Build history of the part. All positions in model axes, mm. Face numbers are marked on the shaded views. A direction names the side the tool comes from. Round coordinates to 2 decimals unless told otherwise and drop trailing zeros. Order: outer loops, then holes, each group sorted by start corner. A loop starts at its lowest first (then second) coordinate and runs counter-clockwise, first axis right, second up. Notation, with made-up numbers: (-32, -16) -> (-25, -16) arc R19 ccw to (-25, 4) -> close; hole circle Ø6 at (-13, 34). An arc over 180 degrees is marked (long way). Write item = value, one per line.
from build123d import *

# Parameters (mm, degrees)
SKETCH1_R           = 0.8
SKETCH1_W           = 15.5
SKETCH1_H           = 10.5
BOSS_EXTRUDE1_DEPTH = 3.8
SKETCH2_R           = 0.8
SKETCH2_W           = 4
SKETCH2_H           = 10.5
BOSS_EXTRUDE2_DEPTH = 1


with BuildPart() as part:
    # Sketch1 → Boss-Extrude1 (new body)
    with BuildSketch(Plane(origin=(0, 0, 0), x_dir=(1, 0, 0), z_dir=(0, 1, 0))):
        with BuildLine():
            Line((-7.75, 6), (7.75, 6))
            ThreePointArc((7.75, 6), (8.62532777, 5.798277313), (9.324082071, 5.233801294))
            Line((9.324082071, 5.233801294), (12.217602589, 1.542251618))
            ThreePointArc((12.217602589, 1.542251618), (12.75, 0), (12.217602589, -1.542251618))
            Line((12.217602589, -1.542251618), (9.324082071, -5.233801294))
            ThreePointArc((9.324082071, -5.233801294), (8.62532777, -5.798277313), (7.75, -6))
            Line((7.75, -6), (-7.75, -6))
            ThreePointArc((-7.75, -6), (-8.62532777, -5.798277313), (-9.324082071, -5.233801294))
            Line((-9.324082071, -5.233801294), (-12.217602589, -1.542251618))
            ThreePointArc((-12.217602589, -1.542251618), (-12.75, 0), (-12.217602589, 1.542251618))
            Line((-12.217602589, 1.542251618), (-9.324082071, 5.233801294))
            ThreePointArc((-9.324082071, 5.233801294), (-8.62532777, 5.798277313), (-7.75, 6))
        make_face()
        with Locations((10.25, 0)):
            Circle(SKETCH1_R, mode=Mode.SUBTRACT)
        with Locations((-10.25, 0)):
            Circle(SKETCH1_R, mode=Mode.SUBTRACT)
        Rectangle(SKETCH1_W, SKETCH1_H, mode=Mode.SUBTRACT)
    extrude(amount=BOSS_EXTRUDE1_DEPTH)

    # Sketch2 → Boss-Extrude2 (add)
    with BuildSketch(Plane(origin=(0, 3.8, 0), x_dir=(1, 0, 0), z_dir=(0, 1, 0))):
        with BuildLine():
            Line((-9.324082071, 5.233801294), (-12.217602589, 1.542251618))
            ThreePointArc((-12.217602589, 1.542251618), (-12.75, 0), (-12.217602589, -1.542251618))
            Line((-12.217602589, -1.542251618), (-9.324082071, -5.233801294))
            ThreePointArc((-9.324082071, -5.233801294), (-8.62532777, -5.798277313), (-7.75, -6))
            Line((-7.75, -6), (7.75, -6))
            ThreePointArc((7.75, -6), (8.62532777, -5.798277313), (9.324082071, -5.233801294))
            Line((9.324082071, -5.233801294), (12.217602589, -1.542251618))
            ThreePointArc((12.217602589, -1.542251618), (12.75, 0), (12.217602589, 1.542251618))
            Line((12.217602589, 1.542251618), (9.324082071, 5.233801294))
            ThreePointArc((9.324082071, 5.233801294), (8.62532777, 5.798277313), (7.75, 6))
            Line((7.75, 6), (-7.75, 6))
            ThreePointArc((-7.75, 6), (-8.62532777, 5.798277313), (-9.324082071, 5.233801294))
        make_face()
        with Locations((10.25, 0)):
            Circle(SKETCH2_R, mode=Mode.SUBTRACT)
        with Locations((-10.25, 0)):
            Circle(SKETCH2_R, mode=Mode.SUBTRACT)
        with Locations((5.75, 0)):
            Rectangle(SKETCH2_W, SKETCH2_H, mode=Mode.SUBTRACT)
    extrude(amount=BOSS_EXTRUDE2_DEPTH)


solid = part.part
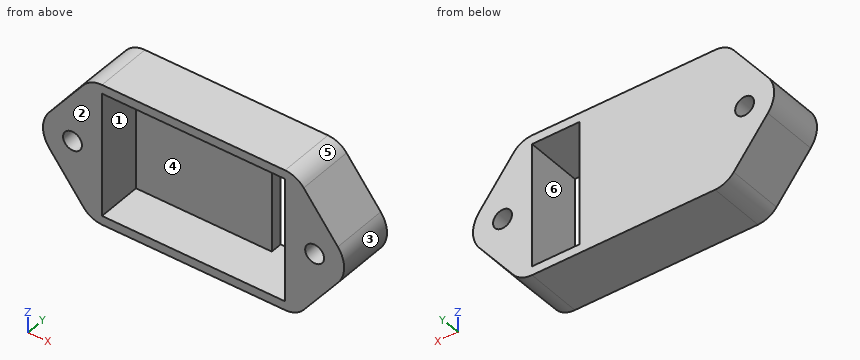
Q1. Cut at D-D, the plane z = 2.25. List the corners of the cut face in (x, y).
Check values:
outline = (-11.66, 0) -> (-7.75, 0) -> (-7.75, 3.8) -> (3.75, 3.8) -> (3.75, 4.8) -> (-11.66, 4.8) -> close; (7.75, 0) -> (11.66, 0) -> (11.66, 4.8) -> (7.75, 4.8) -> close
Q2. Cut at B-B, the plane y = 2.4. List the corners of the cut face in (x, z).
Check values:
outline = (-12.22, -1.54) -> (-9.32, -5.23) arc R2 ccw to (-7.75, -6) -> (7.75, -6) arc R2 ccw to (9.32, -5.23) -> (12.22, -1.54) arc R2.5 ccw to (12.22, 1.54) -> (9.32, 5.23) arc R2 ccw to (7.75, 6) -> (-7.75, 6) arc R2 ccw to (-9.32, 5.23) -> (-12.22, 1.54) arc R2.5 ccw to start; hole circle Ø1.6 at (-10.25, 0); hole (-7.75, -5.25) -> (7.75, -5.25) -> (7.75, 5.25) -> (-7.75, 5.25) -> close; hole circle Ø1.6 at (10.25, 0)
Q3. Cut at A-A, the plane z = 0. List the corners of the cut face in (x, y).
Check values:
outline = (-12.75, 0) -> (-11.05, 0) -> (-11.05, 4.8) -> (-12.75, 4.8) -> close; (-9.45, 0) -> (-7.75, 0) -> (-7.75, 3.8) -> (3.75, 3.8) -> (3.75, 4.8) -> (-9.45, 4.8) -> close; (7.75, 0) -> (9.45, 0) -> (9.45, 4.8) -> (7.75, 4.8) -> close; (11.05, 0) -> (12.75, 0) -> (12.75, 4.8) -> (11.05, 4.8) -> close
Q4. Mould opens along X. For the marked faces 1, 2 and 3 say: released by +X, released by -X, zero draft, split by the parting line, or undercut.
Check values:
face_1 = undercut
face_2 = zero draft
face_3 = released by +X
Q5. Flat gauge pins, fed straight in: pin 1 (2 mm diameter, centred on x = 1, z = 3, fed in from -Y); pin 2 (2 mm diameter, centred on y = 3, z = 0.5, fed in from -X). Where does each tip first touch, or does it go through?
Check values:
pin_1 = 3.8
pin_2 = -12.75
Q6. Probe probe 1 along X at (y, z) = (3.85, 0); probe 2 along X at (y, z) = (1.25, 0); probe 3 along Z at (x, y) = (5.5, 2.1). List the from-to ranges inside material, lowest first.
Check values:
probe_1 = -12.75 to -11.05, -9.45 to 3.75, 7.75 to 9.45, 11.05 to 12.75
probe_2 = -12.75 to -11.05, -9.45 to -7.75, 7.75 to 9.45, 11.05 to 12.75
probe_3 = -6 to -5.25, 5.25 to 6
Q7. Cut at C-C, the plane x = -7. List the corners of the cut face in (y, z), and give its area (3 significant figures).
Check values:
outline = (0, -6) -> (4.8, -6) -> (4.8, 6) -> (0, 6) -> (0, 5.25) -> (3.8, 5.25) -> (3.8, -5.25) -> (0, -5.25) -> close
area = 17.7 mm²
Q8. Which spindle directions (+Z, -Z, +X, -X, +Y, -Y) get a long thin tool onto all of the face, cutting with end or side? Do the marked faces 4, 5 and 6. Say none if no direction does.
Check values:
face_4 = -Y
face_5 = +Z, +X, +Y, -Y
face_6 = +Y, -Y
